```python
from build123d import *

# Parameters (mm, degrees)
SKETCH1_R           = 5.08
SKETCH1_R_2         = 3.556
BOSS_EXTRUDE1_DEPTH = 6.35
SKETCH2_R           = 1.651
CUT_EXTRUDE1_DEPTH  = 6.35
FILLET1_R           = 0.0254


with BuildPart() as part:
    # Sketch1 → Boss-Extrude1 (new body)
    # profile 1 of 2: a face of its own
    with BuildSketch(Plane(origin=(0, 0, 0), x_dir=(1, 0, 0), z_dir=(0, 1, 0))):
        Circle(SKETCH1_R)
        with Locations(Location((0, 0, 0), (0, 0, 270))):
            Circle(SKETCH1_R_2, mode=Mode.SUBTRACT)
    # profile 2 of 2: a face of its own
    with BuildSketch(Plane(origin=(0, 0, 0), x_dir=(1, 0, 0), z_dir=(0, 1, 0))):
        with BuildLine():
            Line((17.664907311, -7.804824457), (10.3349883, -0.769350962))
            Line((10.3349883, -0.769350962), (2.811937974, 4.230768822))
            ThreePointArc((2.811937974, 4.230768822), (3.21777664, 3.93094308), (3.5918694, 3.592335482))
            Line((3.5918694, 3.592335482), (10.264633565, -0.842650153))
            Line((10.264633565, -0.842650153), (17.594552576, -7.878123647))
            Line((17.594552576, -7.878123647), (17.664907311, -7.804824457))
        make_face()
    extrude(amount=BOSS_EXTRUDE1_DEPTH)

    # Sketch2 → Cut-Extrude1 (cut)
    with BuildSketch(Plane(origin=(3.836508416, 0, -5.468082617), x_dir=(-0.7214487215857361, 0, -0.6924678636025697), z_dir=(0.6924678636025697, 0, -0.7214487215857361))):
        with Locations((-15.35754231, 3.175)):
            Circle(SKETCH2_R)
    extrude(amount=-CUT_EXTRUDE1_DEPTH, mode=Mode.SUBTRACT)

    # Fillet1
    fillet1_edges = [part.edges().sort_by_distance(p)[0] for p in [
        (3.5918694, 3.175, -3.592335482),
    ]]
    fillet(fillet1_edges, radius=FILLET1_R)


solid = part.part
```
Build history of the part. All positions in model axes, mm. Give positions to 0.01 mm unless a question says otherwise; leave off trailing zeros. Loops run counter-clockwise (first coordinate to the right, second up) from the corner with the lowest first, then second, coordinate; pieces in that order, holes last.
1) Probe line 1 along X through (y, z) = (4.5, 0.75); line 2 along X through (y, z) = (1.5, 0); line 3 along Z through (x, y) = (1.5, 1.5). List the from-to ranges inside material, lowest first.
Values follow:
line 1: x = -5.02 to -3.48, 3.48 to 5.02, 10.13 to 10.31
line 2: x = -5.08 to -3.56, 3.56 to 5.08, 9 to 9.18
line 3: z = -4.85 to -3.22, 3.22 to 4.85
2) Band-saw the part on C-C on z = -3. List the corners of the cut face in (x, y), then the cut area to 3 significant figures.
Values follow:
outline: (-4.1, 0) - (-1.91, 0) - (-1.91, 6.35) - (-4.1, 6.35) - close; (1.91, 0) - (4.1, 0) - (4.1, 6.35) - (1.91, 6.35) - close; (4.48, 0) - (4.66, 0) - (4.66, 6.35) - (4.48, 6.35) - close
area: 29.0 mm2
3) Band-saw the part on A-A on x = 0. List the corners of the cut face in (y, z), then the cut area to 3 significant figures.
Values follow:
outline: (0, -5.08) - (6.35, -5.08) - (6.35, -3.56) - (0, -3.56) - close; (0, 3.56) - (6.35, 3.56) - (6.35, 5.08) - (0, 5.08) - close
area: 19.4 mm2
4) Band-saw the part on D-D on y = 4.5. List the corners of the cut face in (x, z), then the cut area to 3 significant figures.
Values follow:
outline: (2.81, -4.23) - (10.33, 0.77) - (14.21, 4.48) - (14.14, 4.56) - (10.26, 0.84) - (3.78, -3.47) arc R0.03 cw to (3.75, -3.43) arc R5.08 ccw (long way) to start; (15.56, 5.92) - (15.63, 5.85) - (17.66, 7.8) - (17.59, 7.88) - close; hole circle Ø7.11 at (0, 0)
area: 43.0 mm2
5) Band-saw the part on B-B on y = 2.5. List the corners of the cut face in (x, z), then the cut area to 3 significant figures.
Values follow:
outline: (2.81, -4.23) - (10.33, 0.77) - (13.83, 4.12) - (13.76, 4.2) - (10.26, 0.84) - (3.78, -3.47) arc R0.03 cw to (3.75, -3.43) arc R5.08 ccw (long way) to start; (15.93, 6.28) - (16, 6.21) - (17.66, 7.8) - (17.59, 7.88) - close; hole circle Ø7.11 at (0, 0)
area: 42.9 mm2
